Input: dimensioned drawing with shaded views. Units: mm. Origin: part minimum x, y, z. Round coordinates to 2 decimals unless told otherwise and drop trailing zeros. Loops run counter-clockwise (first coordinate to the right, second up) from the corner with the lowest first, then second, coordinate; pieces in that order, holes last. Notation, with made-up numbers: M -2,29.25 L 20,29.25 A23 ccw 20,55.25 Z; hole C 67,41 d10. An arc over 180 degrees is marked long. Return JSON: item names as keys, results as strings.
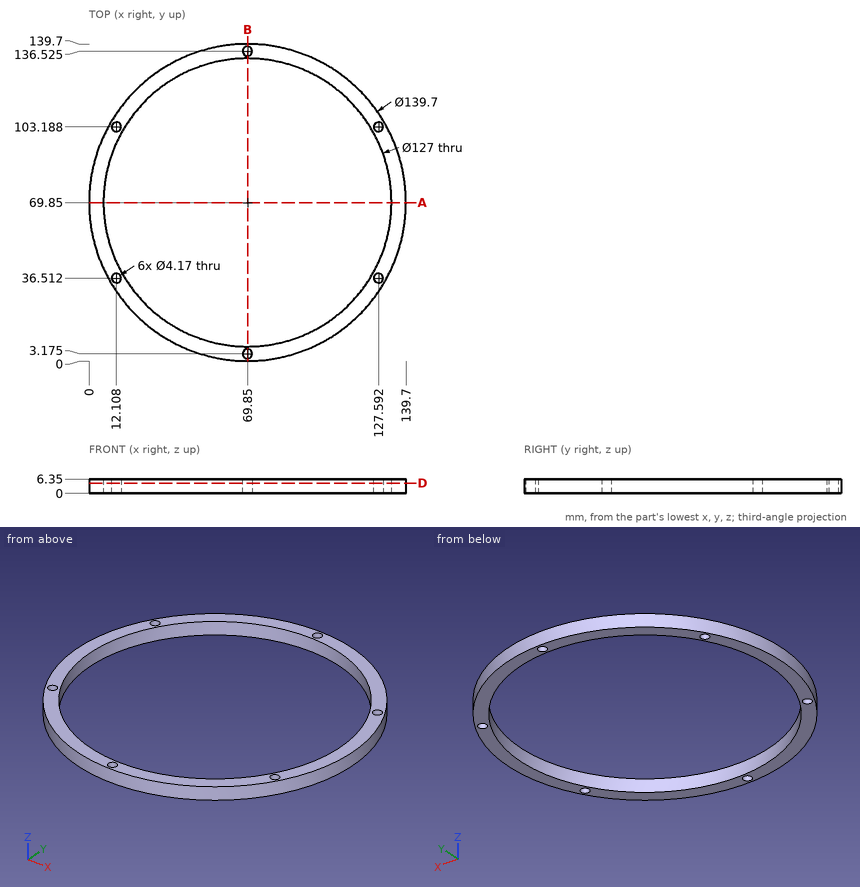
Q1. Section query B-B (x = 69.85). Output: boundary loops of the cut face in (y, z).
Determined:
{"outline": "M 0,0 L 1.09,0 L 1.09,6.35 L 0,6.35 Z; M 5.26,0 L 6.35,0 L 6.35,6.35 L 5.26,6.35 Z; M 133.35,0 L 134.44,0 L 134.44,6.35 L 133.35,6.35 Z; M 138.61,0 L 139.7,0 L 139.7,6.35 L 138.61,6.35 Z"}
Q2. Section query A-A (y = 69.85). Output: boundary loops of the cut face in (x, z).
Determined:
{"outline": "M 0,0 L 6.35,0 L 6.35,6.35 L 0,6.35 Z; M 133.35,0 L 139.7,0 L 139.7,6.35 L 133.35,6.35 Z"}
Q3. Pin query (flat end, axial travel): pin 1 (2.5 mm diameter, centred on x = 69.85, y = 136.525, fed in from -Z); pin 2 (1.5 mm diameter, centred on x = 47, z = 2, fed in from +Y); pin 3 (2 mm diameter, centred on y = 86, z = 2.5, fed in from +X). Return the tip coordinate at first contact, or that it passes through.
Determined:
{"pin 1": "passes through", "pin 2": "stops at y = 136.11", "pin 3": "stops at x = 138.04"}
Q4. Material intervals for L1, parallel to Y at x = 69.85, z = 3.5; L2, parallel to Y at x = 13, z = 6 (1 decimal); L3, parallel to X at y = 105, z = 5.5 (1 decimal), sorted ascending.
Determined:
{"L1": "y = 0 to 1.09, 5.26 to 6.35, 133.35 to 134.44, 138.61 to 139.7", "L2": "y = 29.3 to 34.6, 38.4 to 41.6, 98.1 to 101.3, 105.1 to 110.4", "L3": "x = 9.5 to 11.1, 13.1 to 17, 122.7 to 126.6, 128.6 to 130.2"}
Q5. Section query D-D (z = 4.5). State how many separate pieces and enclosed holes the cut face has, plus the area to 3 significant figures.
Determined:
{"separate pieces": "1", "enclosed holes": "7", "area": "2,580 mm^2"}
